Geometry: see drawing. Coordinates: mm, zero at the bounding-box minimum. Give positions to 0.01 mm unless a question says otherwise; leave off trailing zeros. Loops run counter-clockwise (first coordinate to the right, second up) from the corner with the lowest first, then second, coordinate; pieces in that order, holes last. Notation, with made-up numbers: M 29,13.5 L 75,13.5 A21 ccw 75,41.5 Z; hole C 25.5,67 d7. An arc over 180 degrees is marked long. Answer in a Markdown table with one row per item.
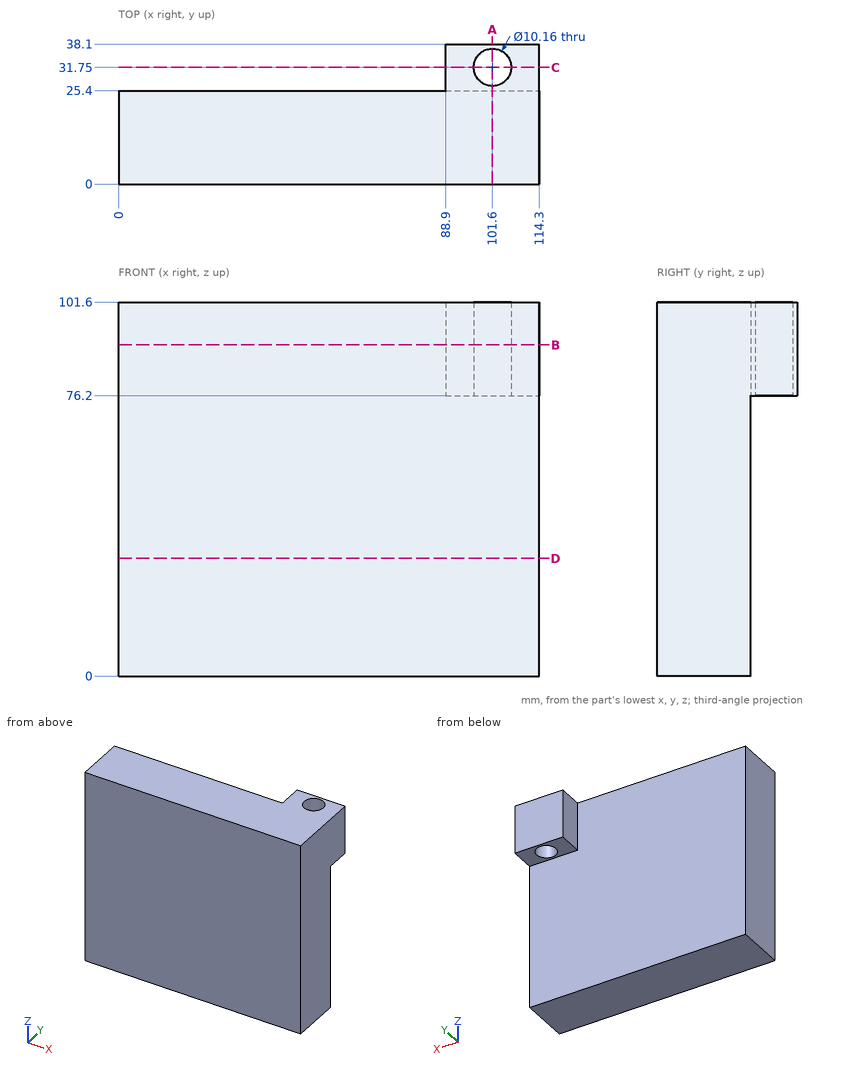
1) Pin query (flat end, axial travel): pin 1 Ø10 at (x, z) = (29.5, 47.5) entering from +Y; pin 2 Ø6.5 at (x, y) = (108, 33.5) entering from -Z; pin 3 Ø6.5 at (y, z) = (30.5, 86.5) entering from -X. Return the tip coordinate at first contact, or that it passes through.
Reply:
| item | result |
|---|---|
| pin 1 | stops at y = 25.4 |
| pin 2 | stops at z = 76.2 |
| pin 3 | stops at x = 88.9 |
2) Material intervals for L1, parallel to Y at x = 101.6, z = 96.25; L2, parallel to X at y = 35, z = 89; L3, parallel to Y at x = 46.5, z = 83.5, sorted ascending.
Reply:
| item | result |
|---|---|
| L1 | y = 0 to 26.67, 36.83 to 38.1 |
| L2 | x = 88.9 to 97.7, 105.5 to 114.3 |
| L3 | y = 0 to 25.4 |
3) Section C-C, the plane y = 31.75. Return loops of the section in (x, z).
Reply:
| item | result |
|---|---|
| outline | M 88.9,76.2 L 96.52,76.2 L 96.52,101.6 L 88.9,101.6 Z; M 106.68,76.2 L 114.3,76.2 L 114.3,101.6 L 106.68,101.6 Z |
4) Section A-A, the plane x = 101.6. Return loops of the section in (y, z), then the cut area to 3 significant figures.
Reply:
| item | result |
|---|---|
| outline | M 0,0 L 25.4,0 L 25.4,76.2 L 26.67,76.2 L 26.67,101.6 L 0,101.6 Z; M 36.83,76.2 L 38.1,76.2 L 38.1,101.6 L 36.83,101.6 Z |
| area | 2,650 mm² |
5) Section B-B, the plane z = 90. Return loops of the section in (x, y), then the cut area to 3 significant figures.
Reply:
| item | result |
|---|---|
| outline | M 0,0 L 114.3,0 L 114.3,38.1 L 88.9,38.1 L 88.9,25.4 L 0,25.4 Z; hole C 101.6,31.75 d10.16 |
| area | 3,140 mm² |
6) Section D-D, the plane z = 32. Return loops of the section in (x, y).
Reply:
| item | result |
|---|---|
| outline | M 0,0 L 114.3,0 L 114.3,25.4 L 0,25.4 Z |
